Work out the finished part from the listing and answer in its coordinate system (mm). A direction names the side the tool comes from. Coordinates: 2 decimals unless noted, no trailing zeros. Loops run counter-clockwise (first coordinate to the right, second up) from the corner with the lowest first, then second, coordinate; pieces in that order, holes last. Notation, with made-up numbers: (50, -2) - (101, -2) arc R22 ccw to (101, 12) - close; hole circle Ø4 at (48.5, 28.5). An arc over 180 degrees is marked (long way). Write each question's results on one line, items separated by ' | '. Start each with the question number.
1. Find the intervals of material crossed by line 1 along Y through (x, z) = (-63.5, -0.65); line 2 along X through (y, z) = (-8, 0.25); line 3 along X through (y, z) = (-10.5, 1.85), in increasing order. Write a range as [from, to].
2. A cutting plane is placed at B-B on x = 63.5. Determine the outline of the cut face in (y, z), then the cut area to 3 significant figures.
3. Each of these flat-tipped pins is pushed along its axis until it touches: P1, Ø2.5, axis at x = 63.5, y = 7.5, coming from the +Z side; P2, Ø1.2, axis at x = 82, z = 1, coming from the -Y side; P3, Ø1.2, axis at y = -7, z = 0.5, coming from the +X side. Where does it stop, or does it pass through?
4. A cutting plane is placed at A-A on y = -7.5. Determine the outline of the cut face in (x, z).
5. Which of the six approach directions +Z, -Z, +X, -X, +Y, -Y give full straight-line access (tool end or side, diameter ignored) to faces 4 (the flat face through (73.5, -7, 0)), 5 (the cylindrical face through (-62.02, 6.89, 0.03))?
6. A cutting plane is placed at C-C on z = -0.7. Determine the outline of the cut face in (x, y), then the cut area to 3 significant figures.
7. A cutting plane is placed at D-D on x = 81.5. Determine the outline of the cut face in (y, z).
8. Determine the mould class of faces 1 (the flat face through (92.5, 10, 0)), 2 (the flat face through (8, 17.5, 0)), 3 (the cylindrical face through (-61.497, -6.869, -0.986)) for opening direction Y: released by +Y, released by -Y, zero draft, split by the parting line, or undercut.
from build123d import *

# Parameters (mm, degrees)
SKETCH_1_W          = 147
SKETCH_1_H          = 35
EXTRUDE_1_DEPTH     = 2
SKETCH_2_W          = 19
SKETCH_2_H          = 15
EXTRUDE_2_DEPTH     = 4
SKETCH_3_R          = 2.1
CUT_EXTRUDE_1_DEPTH = 95.225792647
CHAMFER_1_SIZE      = 4
SKETCH_4_R          = 1
CUT_EXTRUDE_2_DEPTH = 95.225792647
SKETCH_5_R          = 1.6
CUT_EXTRUDE_3_DEPTH = 95.225792647
CHAMFER_2_SIZE      = 2


with BuildPart() as part:
    # 草图1 → 凸台-拉伸1 (new, symmetric)
    with BuildSketch(Plane.XY):
        Rectangle(SKETCH_1_W, SKETCH_1_H)
    extrude(amount=EXTRUDE_1_DEPTH, both=True)

    # 草图2 → 凸台-拉伸2 (add)
    with BuildSketch(Plane.XY.offset(2)):
        with Locations((83, 10)):
            Rectangle(SKETCH_2_W, SKETCH_2_H)
    extrude(amount=-EXTRUDE_2_DEPTH)

    # 草图3 → 切除-拉伸1 (cut, through all)
    with BuildSketch(Plane.XY.offset(2)):
        with Locations((-63.5, -7.5)):
            Circle(SKETCH_3_R)
        with Locations((63.5, -7.5)):
            Circle(SKETCH_3_R)
    extrude(amount=-CUT_EXTRUDE_1_DEPTH, mode=Mode.SUBTRACT)

    # 倒角1
    chamfer_1_edges = [part.edges().sort_by_distance(p)[0] for p in [
        (92.5, 17.5, 0),
        (92.5, 2.5, 0),
        (-73.5, 17.5, 0),
        (73.5, -17.5, 0),
    ]]
    chamfer(chamfer_1_edges, length=CHAMFER_1_SIZE)

    # 草图4 → 切除-拉伸2 (cut, through all)
    with BuildSketch(Plane.XY.offset(2)):
        with Locations((73.5, 1.5)):
            Circle(SKETCH_4_R)
    extrude(amount=-CUT_EXTRUDE_2_DEPTH, mode=Mode.SUBTRACT)

    # 草图5 → 切除-拉伸3 (cut, through all)
    with BuildSketch(Plane.XY.offset(2)):
        with Locations((-63.5, 7.5)):
            Circle(SKETCH_5_R)
        with Locations((-21.166666667, 7.5)):
            Circle(SKETCH_5_R)
        with Locations((21.166666667, 7.5)):
            Circle(SKETCH_5_R)
        with Locations((63.5, 7.5)):
            Circle(SKETCH_5_R)
    extrude(amount=-CUT_EXTRUDE_3_DEPTH, mode=Mode.SUBTRACT)

    # 倒角2
    chamfer_2_edges = [part.edges().sort_by_distance(p)[0] for p in [
        (-65.6, -7.5, 2),
        (61.4, -7.5, 2),
    ]]
    chamfer(chamfer_2_edges, length=CHAMFER_2_SIZE)


solid = part.part
Values:
1) line 1: [-17.5, -9.6], [-5.4, 5.9], [9.1, 17.5] | line 2: [-73.5, -65.8], [-61.2, 61.2], [65.8, 73.5] | line 3: [-73.5, -66.07], [-60.93, 60.93], [66.07, 73.5]
2) outline: (-17.5, -2) - (-9.6, -2) - (-9.6, 0) - (-11.6, 2) - (-17.5, 2) - close; (-5.4, -2) - (5.9, -2) - (5.9, 2) - (-3.4, 2) - (-5.4, 0) - close; (9.1, -2) - (17.5, -2) - (17.5, 2) - (9.1, 2) - close | area: 106 mm^2
3) P1: through | P2: y = 2.5 | P3: x = 73.5
4) outline: (-73.5, -2) - (-65.6, -2) - (-65.6, 0) - (-67.6, 2) - (-73.5, 2) - close; (-61.4, -2) - (61.4, -2) - (61.4, 0) - (59.4, 2) - (-59.4, 2) - (-61.4, 0) - close; (65.6, -2) - (73.5, -2) - (73.5, 2) - (67.6, 2) - (65.6, 0) - close
5) face 4: +Z, -Z, +X, -Y | face 5: +Z, -Z
6) outline: (-73.5, -17.5) - (69.5, -17.5) - (73.5, -13.5) - (73.5, 0.5) arc R1 cw to (73.5, 2.5) - (88.5, 2.5) - (92.5, 6.5) - (92.5, 13.5) - (88.5, 17.5) - (-69.5, 17.5) - (-73.5, 13.5) - close; hole circle Ø4.2 at (-63.5, -7.5); hole circle Ø3.2 at (-63.5, 7.5); hole circle Ø3.2 at (-21.17, 7.5); hole circle Ø3.2 at (21.17, 7.5); hole circle Ø4.2 at (63.5, -7.5); hole circle Ø3.2 at (63.5, 7.5) | area: 5,340 mm^2
7) outline: (2.5, -2) - (17.5, -2) - (17.5, 2) - (2.5, 2) - close
8) face 1: zero draft | face 2: released by +Y | face 3: undercut
